from build123d import *

# Parameters (mm, degrees)
SKICA1_W                 = 1.6
SKICA1_H                 = 0.85
P_IDAT_VYSUNUT_M1_DEPTH  = 0.45
SKICA2_W                 = 6
SKICA2_H                 = 15.5
P_IDAT_VYSUNUT_M2_DEPTH  = 1.5
P_IDAT_START             = 11.5
SKICA4_W                 = 0.6
SKICA4_H                 = 0.6
P_IDAT_VYSUNUT_M4_DEPTH  = 3.6
SKICA6_W                 = 1.6
SKICA6_H                 = 0.85
ODEBRAT_VYSUNUT_M1_DEPTH = 0.45


with BuildPart() as part:
    # Skica1 → Přidat vysunutím1 (new body)
    with BuildSketch(Plane.XY):
        Rectangle(SKICA1_W, SKICA1_H)
    extrude(amount=P_IDAT_VYSUNUT_M1_DEPTH)

    # Skica2 → Přidat vysunutím2 (add)
    with BuildSketch(Plane(origin=(0, 0, 0), x_dir=(-1, 0, 0), z_dir=(0, 0, -1))):
        with Locations((-0.062287775, 4.825)):
            Rectangle(SKICA2_W, SKICA2_H)
    extrude(amount=P_IDAT_VYSUNUT_M2_DEPTH)

    # Skica4 → Přidat vysunutím4 (add)
    with BuildSketch(Plane(origin=(0, 0, 0), x_dir=(1, 0, 0), z_dir=(0, 1, 0)).offset(P_IDAT_START)):
        with Locations((-2.068992039, -0.3)):
            Rectangle(SKICA4_W, SKICA4_H)
        with Locations((2.299906713, -0.3)):
            Rectangle(SKICA4_W, SKICA4_H)
    extrude(amount=P_IDAT_VYSUNUT_M4_DEPTH)

    # Skica6 → Odebrat vysunutím1 (cut)
    with BuildSketch(Plane.XY.offset(0.45)):
        Rectangle(SKICA6_W, SKICA6_H)
    extrude(amount=-ODEBRAT_VYSUNUT_M1_DEPTH, mode=Mode.SUBTRACT)


solid = part.part
For this review, take the finished solid that the model builds, in its own axes (mm). A direction names the side the tool comes from. Give positions to 0.01 mm unless a question says otherwise; leave off trailing zeros. Loops run counter-clockwise (first coordinate to the right, second up) from the corner with the lowest first, then second, coordinate; pieces in that order, holes last. Notation, with made-up numbers: M 25,83.25 L 81,83.25 A28 cw 81,101.25 Z; hole C -13,82 d2. An arc over 180 degrees is marked long. Answer as a JSON object with one key per item and string values. Group by question number.
Q1. Insertion check: P1, Ø0.5, axis at x = -2, y = 14, coming from the -Z side; P2, Ø0.5, axis at y = 14, z = 0.5, coming from the +X side; P3, Ø0.8, axis at x = 1, z = -0.5, coming from the +Y side (3 decimals). Each pin has a flat end and moves straight along its axis. Give the tip position at first contact, or say it passes through.
Q2. Add section C-C on x = 0.3. Give the boundary of the cut face in (y, z) (3 decimals).
Q3. Tool access review of faces 1 (the flat face through (-2.938, 5, -1)), 2 (the flat face through (0, 12.575, -1)): name each direction out of +Z, -Z, +X, -X, +Y, -Y from which nothing blocks a thin tool from reaching the whole face with its end or side.
Q4. Add section B-B on y = 12.25. Give the boundary of the cut face in (x, z).
Q5. Add section A-A on z = 0.2. Give the boundary of the cut face in (x, y), and give its area (3 significant figures).
Q6. For probe 1 along Z at (x, y) = (1.65, 1); probe 2 along Y at (x, z) = (2.2, -0.25) (3 decimals); probe 3 along Z at (x, y) = (2.35, 14), list the stretches that pass through material, from the lowest coordinate up. Write a range as [from, to].
Q7. Add section D-D on y = 7.25. Give the boundary of the cut face in (x, z).
Checked values:
{
 "1": {"P1": "z = 0", "P2": "x = 2.6", "P3": "y = 12.575"},
 "2": {"outline": "M -2.925,-1.5 L 12.575,-1.5 L 12.575,0 L -2.925,0 Z"},
 "3": {"face 1": "+Z, -Z, -X, +Y, -Y", "face 2": "-Z, +X, -X, +Y"},
 "4": {"outline": "M -2.94,-1.5 L 3.06,-1.5 L 3.06,0 L 2.6,0 L 2.6,0.6 L 2,0.6 L 2,0 L -1.77,0 L -1.77,0.6 L -2.37,0.6 L -2.37,0 L -2.94,0 Z"},
 "5": {"outline": "M -2.37,11.5 L -1.77,11.5 L -1.77,15.1 L -2.37,15.1 Z; M 2,11.5 L 2.6,11.5 L 2.6,15.1 L 2,15.1 Z", "area": "4.32 mm²"},
 "6": {"probe 1": "[-1.5, 0]", "probe 2": "[-2.925, 12.575]", "probe 3": "[0, 0.6]"},
 "7": {"outline": "M -2.94,-1.5 L 3.06,-1.5 L 3.06,0 L -2.94,0 Z"}
}
